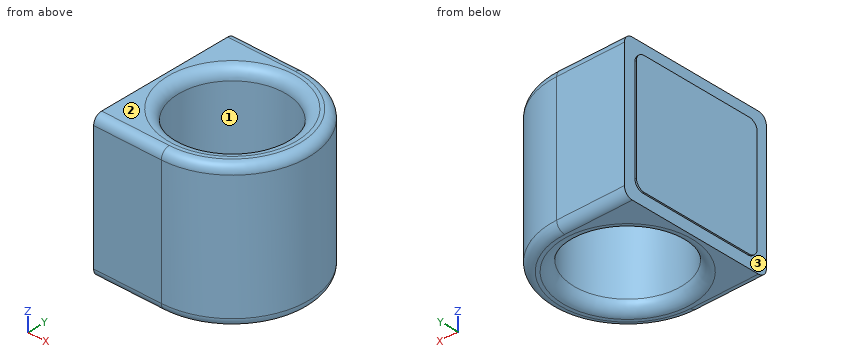
from build123d import *

# Parameters (mm, degrees)
F0_R     = 5.35
F0_R_2   = 3.75
F1_DEPTH = 10
F2_W     = 10.7
F2_H     = 10
F3_DEPTH = 4.75
F4_W     = 7.811706725
F4_H     = 10
F5_DEPTH = 25
F6_DEPTH = 25
F7_W     = 9.1
F7_H     = 8.4
F8_DEPTH = 0.1
F9_R     = 0.6
F10_R    = 0.75


with BuildPart() as f1:
    # F0 (on Top) → F1 (new body)
    with BuildSketch(Plane.XY):
        Circle(F0_R)
        Circle(F0_R_2, mode=Mode.SUBTRACT)
        Circle(F0_R_2)
    extrude(amount=F1_DEPTH)

    # F2 (on Right) → F3 (join)
    with BuildSketch(Plane.YZ):
        with Locations((0, 5)):
            Rectangle(F2_W, F2_H)
    extrude(amount=-F3_DEPTH)

    # F4 (on face) → F5 (cut)
    with BuildSketch(Plane(origin=(-4.75, 0, 0), x_dir=(0, -1, 0), z_dir=(-1, 0, 0))):
        with Locations((1.4441466375, 5)):
            Rectangle(F4_W, F4_H)
    extrude(amount=F5_DEPTH, mode=Mode.SUBTRACT)

    # F0 (on Top) → F6 (cut)
    with BuildSketch(Plane.XY):
        Circle(F0_R_2)
    extrude(amount=F6_DEPTH, mode=Mode.SUBTRACT)

    # F7 (on face) → F8 (join)
    with BuildSketch(Plane(origin=(-4.75, 0, 0), x_dir=(0, -1, 0), z_dir=(-1, 0, 0))):
        with Locations((0, 5)):
            Rectangle(F7_W, F7_H)
    extrude(amount=F8_DEPTH)

    # F9
    f9_edges = [f1.edges().sort_by_distance(p)[0] for p in [
        (-2.375, 5.35, 10),
        (-2.375, 5.35, 0),
        (-2.375, -5.35, 0),
        (-2.375, -5.35, 10),
        (-4.8, 4.55, 9.2),
        (-4.8, -4.55, 9.2),
        (-4.8, -4.55, 0.8),
        (-4.8, 4.55, 0.8),
    ]]
    fillet(f9_edges, radius=F9_R)

    # F10
    f10_edges = [f1.edges().sort_by_distance(p)[0] for p in [
        (-3.75, 0, 0),
        (-3.75, 0, 10),
    ]]
    fillet(f10_edges, radius=F10_R)


solid = f1.part
Input: part model. Units: mm. Frame: model coordinates. Face numbers are marked on the shaded views. Give positions to 0.01 mm unless a question says otherwise; leave off trailing zeros. Write each loop counter-clockwise with the first axis right and the second up, starting at its lowest first coordinate (ties: lowest second). Pieces come first, ordered by that corner, then holes. Notation, with made-up numbers: M 9.5,18 L 21.5,18 A20 ccw 21.5,27 Z; hole C 45,-13 d6. An arc over 180 degrees is marked long. Write item = value, one per line. Start each with the question number.
1) Cut plane A-A on y = 0. Return the cut outline in (x, z), then the cut area to 3 significant figures.
2) First-contact query: pin 1 Ø1 at (x, z) = (1, 2.5) entering from -Y; pin 2 Ø2 at (y, z) = (-2.5, 2.5) entering from +X. Flat tips, straight axial feed; report the tip coordinate or a pass-through.
3) Cut plane B-B on z = 5.25. Return the cut outline in (x, y).
4) Draft query along X for the marked faces 1, 2 and 3. Return one class per face: +X half, -X half, draft (parallel to the pull), parting line (faces both ways), or undercut.
5) Material intervals for line 1 along X through (y, z) = (0, 4); line 2 along Y through (x, z) = (0, 6); line 3 along X through (y, z) = (-3.25, 0.75), sorted ascending. Write a range as [from, to].
Solved:
q1.outline = M -4.85,0.8 L -4.75,0.8 L -4.75,0 L -4.5,0 A0.75 ccw -3.75,0.75 L -3.75,9.25 A0.75 ccw -4.5,10 L -4.75,10 L -4.75,9.2 L -4.85,9.2 Z; M 3.75,0.75 A0.75 ccw 4.5,0 L 4.75,0 A0.6 ccw 5.35,0.6 L 5.35,9.4 A0.6 ccw 4.75,10 L 4.5,10 A0.75 ccw 3.75,9.25 Z
q1.area = 26.2 mm2
q2.pin_1 = -5.33
q2.pin_2 = 5.14
q3.outline = M -4.85,-4.55 L -4.75,-4.55 L -4.75,-5.35 L 0,-5.35 A5.35 ccw 0,5.35 L -4.75,5.35 L -4.75,4.55 L -4.85,4.55 Z; hole C 0,0 d7.5
q4.face_1 = undercut
q4.face_2 = draft
q4.face_3 = -X half
q5.line_1 = [-4.85, -3.75], [3.75, 5.35]
q5.line_2 = [-5.35, -3.75], [3.75, 5.35]
q5.line_3 = [-4.75, -1.87], [1.87, 4.25]
